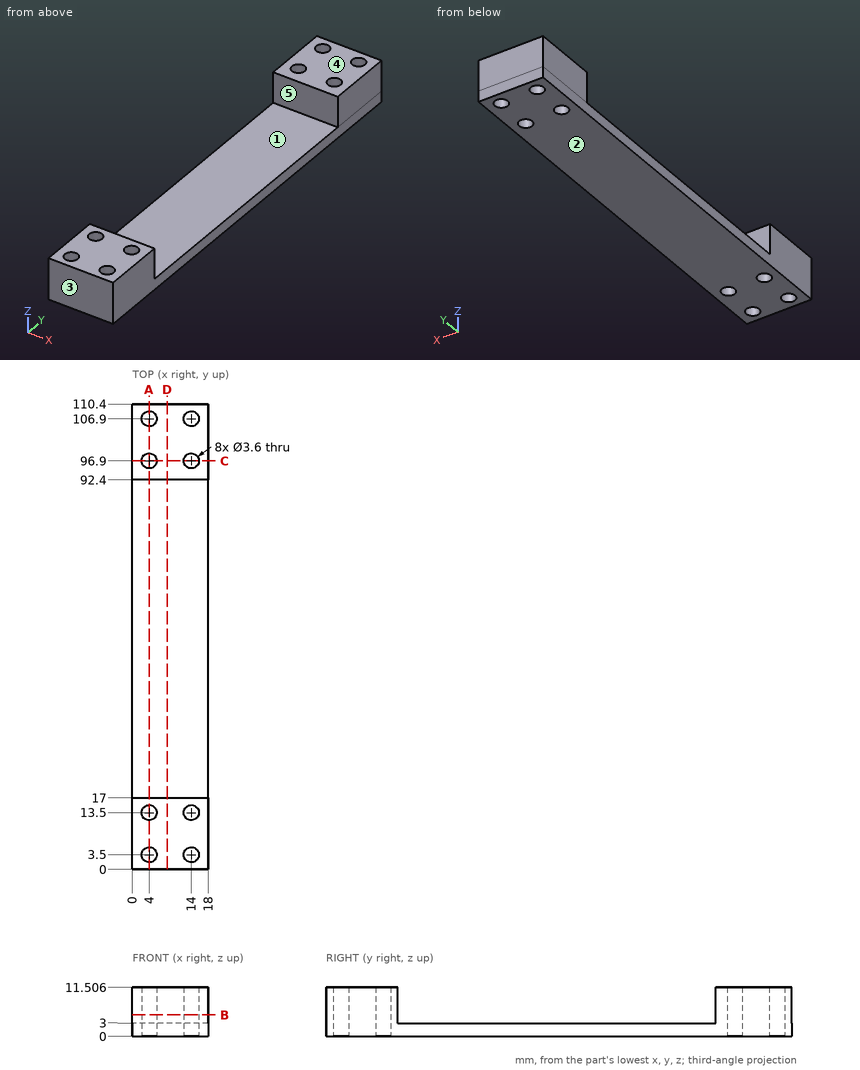
Part print with two shaded views. Sizes in mm from the minimum x, y, z corner. A direction names the side the tool comes from. Coordinates: 2 decimals unless noted, no trailing zeros. Loops run counter-clockwise (first coordinate to the right, second up) from the corner with the lowest first, then second, coordinate; pieces in that order, holes last. Notation, with made-up numbers: (37, 57) - (91, 57) arc R21 ccw to (91, 96) - close; hole circle Ø10 at (74, 74.5). An arc over 180 degrees is marked (long way). Write each question's results on one line, items separated by ' | '. Start each with the question number.
Q1. Which spindle directions (+Z, -Z, +X, -X, +Y, -Y) get a long thin tool onto all of the face, cutting with end or side? Do the marked faces 4 and 5. Say none if no direction does.
Q2. Drop a flat-ended pin along its axis: pin 1 Ø9 at (x, y) = (6, 39) entering from +Z. Give the stop position or say it passes through.
Q3. Two-plate mould, pull along Y, no slides. Class the marked faces 1, 2 and 3: +Y half, -Y half, draft (parallel to the pull), parting line (faces both ways), or undercut.
Q4. Probe line 1 along Y through (x, z) = (4, 5.75); line 2 along X through (y, z) = (96.9, 7); line 3 along Y through (x, z) = (9.25, 10.75). List the from-to ranges inside material, lowest first.
Q5. Slice it at B-B on z = 5. Give the number of separate pieces and of enclosed holes in the cut face.
Q6. Slice it at C-C on y = 96.9. Give the cut face in (x, z) (1 decimal), and give its area (3 significant figures).
Q7. Slice it at A-A on x = 4. Give the cut face in (y, z) (1 decimal).
Q8. Slice it at D-D on x = 8.25. Give the cut face in (y, z) (1 decimal), and give its area (3 significant figures).
Answer:
1) face 4: +Z, +X, -X, +Y, -Y | face 5: +Z, +X, -X
2) pin 1: stops at z = 3
3) face 1: undercut | face 2: draft | face 3: -Y half
4) line 1: y = 0 to 1.7, 5.3 to 11.7, 15.3 to 17, 92.4 to 95.1, 98.7 to 105.1, 108.7 to 110.4 | line 2: x = 0 to 2.2, 5.8 to 12.2, 15.8 to 18 | line 3: y = 0 to 17, 92.4 to 110.4
5) separate pieces: 2 | enclosed holes: 8
6) outline: (0, 0) - (2.2, 0) - (2.2, 11.5) - (0, 11.5) - close; (5.8, 0) - (12.2, 0) - (12.2, 11.5) - (5.8, 11.5) - close; (15.8, 0) - (18, 0) - (18, 11.5) - (15.8, 11.5) - close | area: 124 mm2
7) outline: (0, 0) - (1.7, 0) - (1.7, 11.5) - (0, 11.5) - close; (5.3, 0) - (11.7, 0) - (11.7, 11.5) - (5.3, 11.5) - close; (15.3, 0) - (95.1, 0) - (95.1, 11.5) - (92.4, 11.5) - (92.4, 3) - (17, 3) - (17, 11.5) - (15.3, 11.5) - close; (98.7, 0) - (105.1, 0) - (105.1, 11.5) - (98.7, 11.5) - close; (108.7, 0) - (110.4, 0) - (110.4, 11.5) - (108.7, 11.5) - close
8) outline: (0, 0) - (110.4, 0) - (110.4, 11.5) - (92.4, 11.5) - (92.4, 3) - (17, 3) - (17, 11.5) - (0, 11.5) - close | area: 629 mm2
